```python
from build123d import *

# Parameters (mm, degrees)
CROQUIS1_W              = 20
CROQUIS1_H              = 20
CROQUIS1_R              = 1.55
SALIENTE_EXTRUIR1_DEPTH = 3
CROQUIS2_W              = 20
CROQUIS2_H              = 5
SALIENTE_EXTRUIR3_DEPTH = 15
SALIENTE_EXTRUIR4_DEPTH = 5
SALIENTE_EXTRUIR5_DEPTH = 5
CROQUIS5_R              = 2
CORTAR_EXTRUIR1_DEPTH   = 21


with BuildPart() as part:
    # Croquis1 → Saliente-Extruir1 (new body)
    with BuildSketch(Plane.XY):
        with Locations((10, 10)):
            Rectangle(CROQUIS1_W, CROQUIS1_H)
        with Locations((10, 10)):
            Circle(CROQUIS1_R, mode=Mode.SUBTRACT)
    extrude(amount=-SALIENTE_EXTRUIR1_DEPTH)

    # Croquis2 → Saliente-Extruir3 (add)
    with BuildSketch(Plane.XY):
        with Locations((10, 2.5)):
            Rectangle(CROQUIS2_W, CROQUIS2_H)
        with Locations((10, 17.5)):
            Rectangle(CROQUIS2_W, CROQUIS2_H)
    extrude(amount=SALIENTE_EXTRUIR3_DEPTH)

    # Croquis3 → Saliente-Extruir4 (add)
    with BuildSketch(Plane(origin=(0, 20, 0), x_dir=(1, 0, 0), z_dir=(0, 1, 0))):
        with BuildLine():
            Line((20, -15), (0, -15))
            Line((0, -15), (0, -25))
            Line((0, -25), (10, -25))
            ThreePointArc((10, -25), (17.071067812, -22.071067812), (20, -15))
        make_face()
    extrude(amount=-SALIENTE_EXTRUIR4_DEPTH)

    # Croquis4 → Saliente-Extruir5 (add)
    with BuildSketch(Plane.XZ):
        with BuildLine():
            Line((0, 15), (20, 15))
            ThreePointArc((20, 15), (17.071067812, 22.071067812), (10, 25))
            Line((10, 25), (0, 25))
            Line((0, 25), (0, 15))
        make_face()
    extrude(amount=-SALIENTE_EXTRUIR5_DEPTH)

    # Croquis5 → Cortar-Extruir1 (cut, through all)
    with BuildSketch(Plane.XZ):
        with Locations((10, 15)):
            Circle(CROQUIS5_R)
    extrude(amount=-CORTAR_EXTRUIR1_DEPTH, mode=Mode.SUBTRACT)


solid = part.part
```
Source: CAD feature listing. Evaluate the final solid. Frame: model axes, mm. A direction names the side the tool comes from. Round coordinates to 2 decimals unless told otherwise and drop trailing zeros. Order: outer loops, then holes, each group sorted by start corner. A loop starts at its lowest first (then second) coordinate and runs counter-clockwise, first axis right, second up. Notation, with made-up numbers: (50.5, -28) -> (108.5, -28) arc R7 cw to (108.5, -17) -> close; hole circle Ø4 at (-5, 85). An arc over 180 degrees is marked (long way). One line per item, written item: value. Start each with the question number.
Q1. Draft query along Z for faces 3 (the cylindrical face through (16.99, 17.54, 22.15)), 4 (the flat face through (20, 10, -2)), 5 (the flat face through (12, 10, -3)), 6 (the cylindrical face through (10, 2, 17)). Return one class per face: pulls with the +Z half, pulls with the -Z half, needs draft (parallel to the pull), parting line crosses it, or undercut.
Q2. Section query B-B (y = 10). Return the cut outline in (x, z), plus the area to 3 significant figures.
Q3. Section query C-C (z = 14.25). Return the cut outline in (x, y), plus the area to 3 significant figures.
Q4. Section query D-D (x = 5.25). Return the cut outline in (y, z).
Q5. Section query A-A (z = 3). Return the cut outline in (x, y).
Q6. Pin query (flat end, axial travel): pin 1 (5 mm diameter, centred on x = 7.5, y = 12, fed in from +Z). Return the tip coordinate at first contact, or that it passes through.
Q7. Access query for faces 1 (the flat face through (10, 20, 11)), 2 (the flat face through (12, 10, 0)). Directions: +Z, -Z, +X, -X, +Y, -Y. A direction counts if a zero-diameter tool reaches every point of the face in a straight line with its end or side. Return the directions, or none.
Q8. Material intervals for probe 1 along Y at (x, z) = (7.5, 7.75); probe 2 along Y at (x, z) = (10, -1.15); probe 3 along Z at (x, y) = (10, 3.05), sorted ascending.
Findings below:
1. face 3: pulls with the +Z half
1. face 4: needs draft
1. face 5: pulls with the -Z half
1. face 6: undercut
2. outline: (0, -3) -> (8.45, -3) -> (8.45, 0) -> (0, 0) -> close; (11.55, -3) -> (20, -3) -> (20, 0) -> (11.55, 0) -> close
2. area: 50.7 mm²
3. outline: (0, 0) -> (8.15, 0) -> (8.15, 5) -> (0, 5) -> close; (0, 15) -> (8.15, 15) -> (8.15, 20) -> (0, 20) -> close; (11.85, 0) -> (20, 0) -> (20, 5) -> (11.85, 5) -> close; (11.85, 15) -> (20, 15) -> (20, 20) -> (11.85, 20) -> close
3. area: 163 mm²
4. outline: (0, -3) -> (20, -3) -> (20, 25) -> (15, 25) -> (15, 0) -> (5, 0) -> (5, 25) -> (0, 25) -> close
5. outline: (0, 0) -> (20, 0) -> (20, 5) -> (0, 5) -> close; (0, 15) -> (20, 15) -> (20, 20) -> (0, 20) -> close
6. pin 1: z = 0
7. face 1: +Z, -Z, +X, -X, +Y
7. face 2: +Z, +X, -X
8. probe 1: 0 to 5, 15 to 20
8. probe 2: 0 to 8.45, 11.55 to 20
8. probe 3: -3 to 13, 17 to 25
